Input: part model. Units: mm. Frame: model coordinates. Face numbers are marked on the shaded views. A direction names the side the tool comes from. Round coordinates to 2 decimals unless told otherwise and drop trailing zeros. Write each loop counter-clockwise with the first axis right and the second up, starting at its lowest first coordinate (ties: lowest second). Pieces come first, ordered by that corner, then holes. Notation, with made-up numbers: (84, 25.5) -> (140, 25.5) arc R7 cw to (140, 33.5) -> close; hole circle Ø8 at (69.5, -19). An arc over 180 degrees is marked (long way). Use CSV: the item, a comma, the result in double quotes.
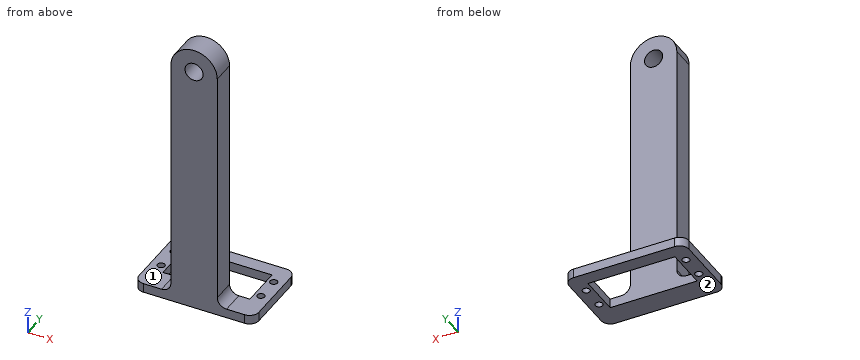
```python
from build123d import *

# Parameters (mm, degrees)
SKETCH1_W           = 12.7
SKETCH1_H           = 6.35
BOSS_EXTRUDE1_DEPTH = 38.1
CUT_EXTRUDE1_REACH  = 41.144
SKETCH2_R           = 2.4765
FILLET1_RADIUS      = 6.35
FILLET1_LENGTH      = 6.35
SKETCH3_W           = 32.7914
SKETCH3_H           = 21.59
SKETCH3_R           = 0.999998
SKETCH3_W_2         = 23.7998
SKETCH3_H_2         = 11.43
BOSS_EXTRUDE2_DEPTH = 2.54
FILLET3_R           = 2.54


with BuildPart() as part:
    # Sketch1 → Boss-Extrude1 (new, symmetric)
    with BuildSketch(Plane.XY):
        Rectangle(SKETCH1_W, SKETCH1_H)
    extrude(amount=BOSS_EXTRUDE1_DEPTH, both=True)

    # Sketch2 → Cut-Extrude1 (cut, up to next)
    with BuildSketch(Plane(origin=(0, 3.175, 0), x_dir=(1, 0, 0), z_dir=(0, 1, 0)), mode=Mode.PRIVATE) as cut_extrude1_sk1:
        with Locations(Location((0, -31.75, 0), (0, 0, 270))):
            Circle(SKETCH2_R)
    cut_extrude1_tool1 = extrude(cut_extrude1_sk1.sketch, amount=-CUT_EXTRUDE1_REACH, mode=Mode.PRIVATE) & part.part
    add(cut_extrude1_tool1.solids().sort_by_distance((0, 3.175, 31.75))[0], mode=Mode.SUBTRACT)

    # Fillet1: full round fillet: the end face becomes a half cylinder, R = half its width
    fillet1_face = Plane((0, 0, 38.1), x_dir=(0, 1, 0), z_dir=(0, 0, 1))  # on the end face: x along it, z out of the body
    fillet1_slab = fillet1_face.offset(-FILLET1_RADIUS / 2) * Box(FILLET1_LENGTH, 2 * FILLET1_RADIUS, FILLET1_RADIUS, mode=Mode.PRIVATE)  # the body's end, R deep
    fillet1_round = Plane((0, 0, 31.75), x_dir=(0, 0, 1), z_dir=(0, 1, 0)) * Cylinder(FILLET1_RADIUS, FILLET1_LENGTH, mode=Mode.PRIVATE)  # its axis R under the face
    add(fillet1_slab - fillet1_round, mode=Mode.SUBTRACT)

    # Sketch3 → Boss-Extrude2 (add)
    with BuildSketch(Plane(origin=(0, 0, -38.1), x_dir=(-1, 0, 0), z_dir=(0, 0, -1))):
        with Locations((0, 7.62)):
            Rectangle(SKETCH3_W, SKETCH3_H)
        with Locations((13.65, 5.588)):
            Circle(SKETCH3_R, mode=Mode.SUBTRACT)
        with Locations((13.65, 12.192)):
            Circle(SKETCH3_R, mode=Mode.SUBTRACT)
        with Locations((-13.65, 5.588)):
            Circle(SKETCH3_R, mode=Mode.SUBTRACT)
        with Locations((-13.65, 12.192)):
            Circle(SKETCH3_R, mode=Mode.SUBTRACT)
        with Locations((0, 8.89)):
            Rectangle(SKETCH3_W_2, SKETCH3_H_2, mode=Mode.SUBTRACT)
    extrude(amount=-BOSS_EXTRUDE2_DEPTH)

    # Fillet3
    fillet3_edges = [part.edges().sort_by_distance(p)[0] for p in [
        (-6.35, 0, -35.56),
        (6.35, 0, -35.56),
        (-16.3957, -3.175, -36.83),
        (16.3957, -3.175, -36.83),
        (16.3957, 18.415, -36.83),
        (-16.3957, 18.415, -36.83),
    ]]
    fillet(fillet3_edges, radius=FILLET3_R)


solid = part.part
```
Item 1: Set-up query: the marked faces 1 and 2. Return all of +Z, -Z, +X, -X, +Y, -Y with unobstructed straight access to the full face (end or side cutting, diameter ignored); none if empty.
Worked answers:
face 1,"+Z, +Y"
face 2,"-Z, +X, -X, +Y, -Y"
Item 2: Section query B-B on z = -26.5. Return the cut outline in (x, y) (3 decimals), plus the area to 3 significant figures.
Worked answers:
outline,"(-6.35, -3.175) -> (6.35, -3.175) -> (6.35, 3.175) -> (-6.35, 3.175) -> close"
area,"80.6 mm²"
Item 3: Line query: line 1 (Y direction, x = 13.65, z = -36.6) (3 decimals); line 2 (Y direction, x = 13, z = -36) (3 decimals); line 3 (Z direction, x = -10, y = 0.25). Output: solid intervals per line, ascending.
Worked answers:
line 1,"y = -3.175 to 4.588, 6.588 to 11.192, 13.192 to 18.415"
line 2,"y = -3.175 to 4.828, 6.348 to 11.432, 12.952 to 18.415"
line 3,"z = -38.1 to -35.56"
Item 4: Section query A-A on x = 0. Return the cut outline in (y, z) (1 decimal), plus the area to 3 significant figures.
Worked answers:
outline,"(-3.2, -38.1) -> (3.2, -38.1) -> (3.2, 29.3) -> (-3.2, 29.3) -> close; (-3.2, 34.2) -> (3.2, 34.2) -> (3.2, 38.1) -> (-3.2, 38.1) -> close; (14.6, -38.1) -> (18.4, -38.1) -> (18.4, -35.6) -> (14.6, -35.6) -> close"
area,"462 mm²"
Item 5: First-contact query: pin 1 Ø8 at (x, z) = (0, 31.75) entering from -Y (3 decimals); pin 2 Ø3 at (y, z) = (0, 5.5) entering from -X; pin 3 Ø1.2 at (x, y) = (13.65, 5.588) entering from +Z; pin 4 Ø3 at (x, y) = (5.5, 16) entering from +Z. Flat tips, straight axial feed; report the tip coordinate or a pass-through.
Worked answers:
pin 1,"stops at y = -3.175"
pin 2,"stops at x = -6.35"
pin 3,"passes through"
pin 4,"stops at z = -35.56"
